Answer from the drawing. Dimensions are ordinates in mm from the lowest x, y and z of the part. Give positions to 0.01 mm unless a question says otherwise; leave off trailing zeros. Write each loop counter-clockwise with the first axis right and the second up, starting at its lowest first coordinate (ties: lowest second). Pieces come first, ordered by that corner, then holes. Notation, with made-up numbers: (18, 14.25) -> (41, 14.25) arc R19 ccw to (41, 21.25) -> close; hole circle Ø9 at (-26.5, -2). An arc over 180 degrees is marked (long way). Put each result on its own line as item: value. Start each with the question number.
1) Find the intervals of material crossed by line 1 along Y through (x, z) = (7, 1); line 2 along Y through (x, z) = (17, 0.4); line 3 along X through (y, z) = (6.75, 1.35), in increasing order. Write a range as from..to.
2) A cutting plane is placed at B-B (x = 17). Write down the section's boundary in (y, z).
3) A cutting plane is placed at D-D (x = 57). Write down the section's boundary in (y, z).
4) A cutting plane is placed at C-C (z = 0.9). Write down the section's boundary in (x, y).
5) A cutting plane is placed at A-A (y = 6.5). Write down the section's boundary in (x, z).
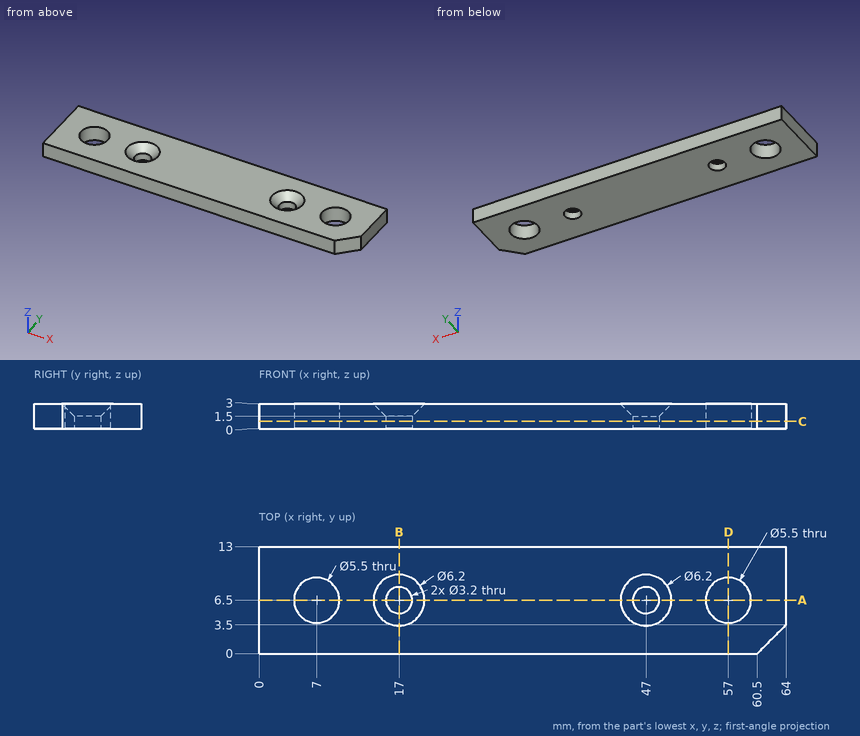
Reply:
1. line 1: y = 0..3.75, 9.25..13
1. line 2: y = 0..4.9, 8.1..13
1. line 3: x = 0..4.26, 9.74..15.42, 18.58..45.42, 48.58..54.26, 59.74..64
2. outline: (0, 0) -> (4.9, 0) -> (4.9, 1.5) -> (3.4, 3) -> (0, 3) -> close; (8.1, 0) -> (13, 0) -> (13, 3) -> (9.6, 3) -> (8.1, 1.5) -> close
3. outline: (0, 0) -> (3.75, 0) -> (3.75, 3) -> (0, 3) -> close; (9.25, 0) -> (13, 0) -> (13, 3) -> (9.25, 3) -> close
4. outline: (0, 0) -> (60.5, 0) -> (64, 3.5) -> (64, 13) -> (0, 13) -> close; hole circle Ø5.5 at (7, 6.5); hole circle Ø3.2 at (17, 6.5); hole circle Ø3.2 at (47, 6.5); hole circle Ø5.5 at (57, 6.5)
5. outline: (0, 0) -> (4.25, 0) -> (4.25, 3) -> (0, 3) -> close; (9.75, 0) -> (15.4, 0) -> (15.4, 1.5) -> (13.9, 3) -> (9.75, 3) -> close; (18.6, 0) -> (45.4, 0) -> (45.4, 1.5) -> (43.9, 3) -> (20.1, 3) -> (18.6, 1.5) -> close; (48.6, 0) -> (54.25, 0) -> (54.25, 3) -> (50.1, 3) -> (48.6, 1.5) -> close; (59.75, 0) -> (64, 0) -> (64, 3) -> (59.75, 3) -> close
